The drawing under review shows one solid part. Ordinate dimensions are in mm from its lowest x, y, z. A direction names the side the tool comes from. Round coordinates to 2 decimals unless told otherwise and drop trailing zeros. Write each loop counter-clockwise with the first axis right and the second up, starting at its lowest first coordinate (ties: lowest second). Pieces come first, ordered by that corner, then holes. Notation, with made-up numbers: M -34,1.5 L 13,1.5 A21 cw 13,35.5 Z; hole C 77,-27.5 d2. An arc over 180 degrees is marked long. One line per item, written item: value. Start each with the question number.
1) Take a section at C-C, the plane z = 6.75. Write out the cut boundary in (x, y).
2) Take a section at B-B, the plane y = 5.25. Write out the cut boundary in (x, z).
3) For P1, Ø1.5, axis at x = 3.5, z = 3.5, coming from the +Y side (1 decimal); P2, Ø1, axis at y = 1, z = 8.5, coming from the -X side; P3, Ø1, axis at x = 5, z = 7, coming from the -Y side; P4, Ø2.5, axis at x = 5, y = 4, coming from the +Z side, all flat-tipped, find the tip position at first contact; note any pin that passes through.
4) Take a section at A-A, the plane x = 5. Write out the cut boundary in (y, z).
5) Mouldability with a two-part tool opening along Z and no side actions: class the marked faces 6, 7, 8 and 9 as +Z half, -Z half, draft (parallel to the pull), parting line (faces both ways), or undercut.
6) Take a section at D-D, the plane y = 3.35. Write out the cut boundary in (x, z).
7) Tool access review of the marked faces 1, 2, 3, 4 and 5: name each direction out of +Z, -Z, +X, -X, +Y, -Y from which nothing blocks a thin tool from reaching the whole face with its end or side.
8) Wall thickness on probe 1 along Z at (x, y) = (6.25, 3.4); probe 2 along Y at (x, z) = (5, 3.15); probe 3 along Y at (x, z) = (9, 7.75): over which ranges is each line inside the solid? List them lowest first.
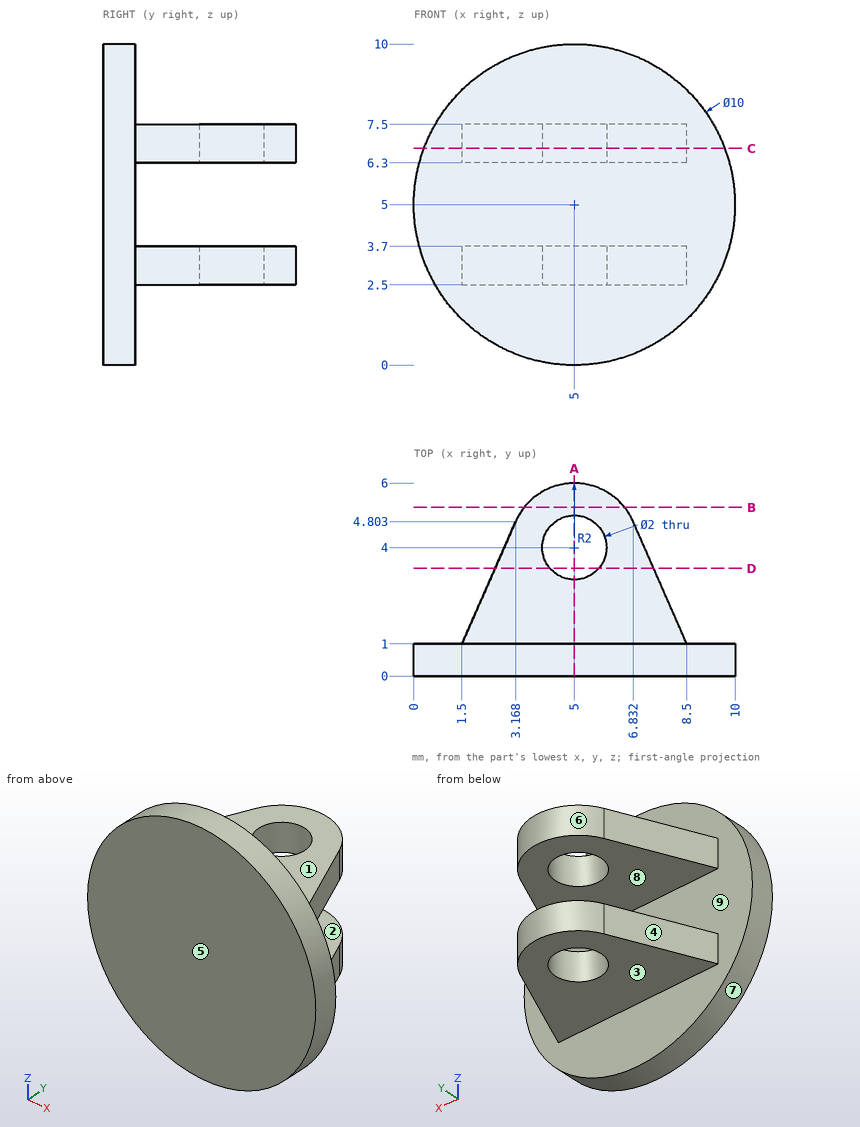
Checked values:
1. outline: M 0.32,0 L 9.68,0 L 9.68,1 L 8.5,1 L 6.83,4.8 A2 ccw 3.17,4.8 L 1.5,1 L 0.32,1 Z; hole C 5,4 d2
2. outline: M 3.44,2.5 L 6.56,2.5 L 6.56,3.7 L 3.44,3.7 Z; M 3.44,6.3 L 6.56,6.3 L 6.56,7.5 L 3.44,7.5 Z
3. P1: stops at y = 5.9
3. P2: stops at x = 1
3. P3: stops at y = 0
3. P4: stops at z = 7.5
4. outline: M 0,0 L 1,0 L 1,2.5 L 3,2.5 L 3,3.7 L 1,3.7 L 1,6.3 L 3,6.3 L 3,7.5 L 1,7.5 L 1,10 L 0,10 Z; M 5,2.5 L 6,2.5 L 6,3.7 L 5,3.7 Z; M 5,6.3 L 6,6.3 L 6,7.5 L 5,7.5 Z
5. face 6: draft
5. face 7: parting line
5. face 8: undercut
5. face 9: undercut
6. outline: M 2.53,2.5 L 4.24,2.5 L 4.24,3.7 L 2.53,3.7 Z; M 2.53,6.3 L 4.24,6.3 L 4.24,7.5 L 2.53,7.5 Z; M 5.76,2.5 L 7.47,2.5 L 7.47,3.7 L 5.76,3.7 Z; M 5.76,6.3 L 7.47,6.3 L 7.47,7.5 L 5.76,7.5 Z
7. face 1: +Z, +X, -X, +Y
7. face 2: +X, -X, +Y
7. face 3: -Z, +X, -X, +Y
7. face 4: +Z, -Z, -X, +Y
7. face 5: +Z, -Z, +X, -X, -Y
8. probe 1: z = 2.5 to 3.7, 6.3 to 7.5
8. probe 2: y = 0 to 3, 5 to 6
8. probe 3: y = 0 to 1
